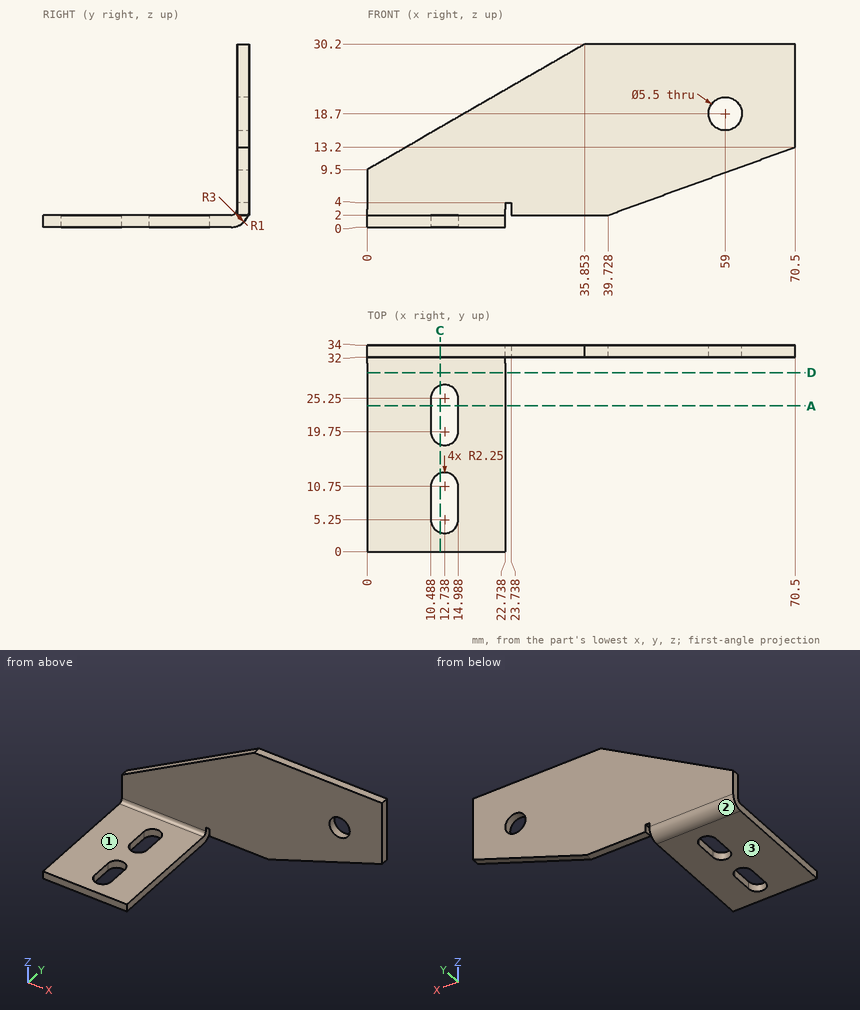
Answer from the drawing. Dimensions are ordinates in mm from the lowest x, y and z of the part. A direction names the side the tool comes from. Coordinates: 2 decimals unless noted, no trailing zeros. Loops run counter-clockwise (first coordinate to the right, second up) from the corner with the lowest first, then second, coordinate; pieces in that order, holes last.
Q1. Consider probe 1 along Y at (x, z) = (66, 13); probe 2 along Z at (x, y) = (6, 11); probe 3 along X at (y, z) = (33, 18) (1 decimal). Determine where each line is inside the solid, lowest interval first.
Q2. The part is cut by section D-D on y = 29.5. Write down the section's boundary in (x, z).
Q3. The part is cut by section C-C on x = 12. Write down the section's boundary in (y, z) (1 decimal).
Q4. Each of these flat-tipped pins is pushed along its axis until it touches: pin 1 Ø4.5 at (y, z) = (11.5, 1.5) entering from +X; pin 2 Ø1.1 at (x, y) = (23.5, 33) entering from -Z; pin 3 Ø3.5 at (x, z) = (59, 18.7) entering from -Y; pin 4 Ø8.5 at (x, z) = (52, 11) entering from -Y. Where does it stop, or does it pass through?
Q5. The part is cut by section A-A on y = 24. Write down the section's boundary in (x, z).
Q6. Which of the six approach directions +Z, -Z, +X, -X, +Y, -Y give full straight-line access (tool end or side, diameter ignored) to the marked faces 1, 2 and 3?
Results below:
1. probe 1: y = 32 to 34
1. probe 2: z = 0 to 2
1. probe 3: x = 14.7 to 56.3, 61.7 to 70.5
2. outline: (0, 0) - (22.74, 0) - (22.74, 2) - (0, 2) - close
3. outline: (0, 0) - (3.1, 0) - (3.1, 2) - (0, 2) - close; (12.9, 0) - (17.6, 0) - (17.6, 2) - (12.9, 2) - close; (27.4, 0) - (31, 0) arc R3 ccw to (34, 3) - (34, 16.4) - (32, 16.4) - (32, 3) arc R1 cw to (31, 2) - (27.4, 2) - close
4. pin 1: stops at x = 22.74
4. pin 2: stops at z = 2
4. pin 3: passes through
4. pin 4: stops at y = 32
5. outline: (0, 0) - (10.49, 0) - (10.49, 2) - (0, 2) - close; (14.99, 0) - (22.74, 0) - (22.74, 2) - (14.99, 2) - close
6. face 1: +Z, +X, -X, -Y
6. face 2: -Z, -X, +Y
6. face 3: -Z, +X, -X, +Y, -Y
